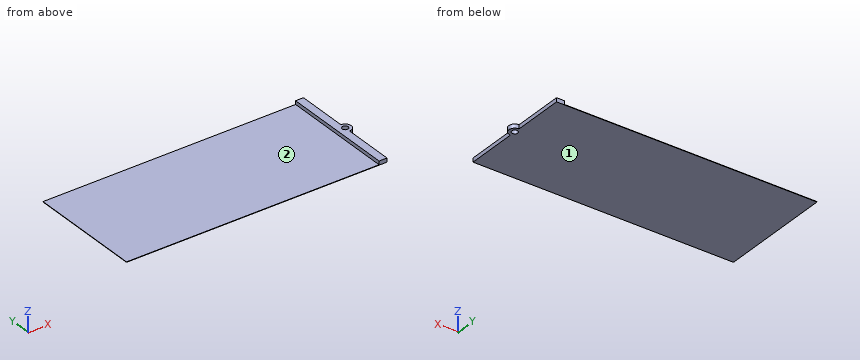
```python
from build123d import *

# Parameters (mm, degrees)
F0_R     = 9.525
F1_DEPTH = 12.7
F2_W     = 812.8
F2_H     = 368.3
F3_DEPTH = 1.27


with BuildPart() as f1:
    # F0 (on Top) → F1 (new body)
    with BuildSketch(Plane.XY):
        with BuildLine():
            Line((-157.734471, -102.348973), (-132.334471, -102.348973))
            Line((-132.334471, -102.348973), (-132.334471, 62.751027))
            ThreePointArc((-132.334471, 62.751027), (-113.284471, 81.801027), (-132.334471, 100.851027))
            Line((-132.334471, 100.851027), (-132.334471, 265.951027))
            Line((-132.334471, 265.951027), (-157.734471, 265.951027))
            Line((-157.734471, 265.951027), (-157.734471, -102.348973))
        make_face()
        with Locations((-132.334471, 81.801027)):
            Circle(F0_R, mode=Mode.SUBTRACT)
    extrude(amount=F1_DEPTH)

    # F2 (on Top) → F3 (join)
    with BuildSketch(Plane.XY):
        with Locations((-564.134471, 81.801027)):
            Rectangle(F2_W, F2_H)
    extrude(amount=F3_DEPTH)


solid = f1.part
```
The listing builds one solid part. Answer for the finished solid, in the listing's coordinates (mm). Face numbers are marked on the shaded views. A direction names the side the tool comes from. Round coordinates to 2 decimals unless told otherwise and drop trailing zeros. Loops run counter-clockwise (first coordinate to the right, second up) from the corner with the lowest first, then second, coordinate; pieces in that order, holes last.
1) A cutting plane is placed at A-A on y = 37.5. Determine the outline of the cut face in (x, z).
Outcome:
outline: (-970.53, 0) - (-132.33, 0) - (-132.33, 12.7) - (-157.73, 12.7) - (-157.73, 1.27) - (-970.53, 1.27) - close
2) A cutting plane is placed at C-C on x = -374. Determine the outline of the cut face in (y, z), plus the area to 3 significant figures.
Outcome:
outline: (-102.35, 0) - (265.95, 0) - (265.95, 1.27) - (-102.35, 1.27) - close
area: 468 mm2
3) Given P1, Ø2, axis at x = -868.5, y = 173, coming from the +Z side; P2, Ø6, axis at x = -595.5, y = -42.5, coming from the -Z side; P3, Ø6, axis at y = 220, z = 4.5, coming from the +X side, each flat-ended and moving along its own axis, determine where each tip first touches the part or whether it passes through.
Outcome:
P1: stops at z = 1.27
P2: stops at z = 0
P3: stops at x = -132.33
4) Consider line 1 (X direction, y = 83, z = 12.25); line 2 (X direction, y = 109.5, z = 12.25); line 3 (Z direction, x = -698, y = 103). Determine where each line is inside the solid, lowest interval first.
Outcome:
line 1: x = -157.73 to -141.78, -122.89 to -113.32
line 2: x = -157.73 to -132.33
line 3: z = 0 to 1.27
5) A cutting plane is placed at B-B on z = 8.5. Determine the outline of the cut face in (x, y) (3 decimals).
Outcome:
outline: (-157.734, -102.349) - (-132.334, -102.349) - (-132.334, 62.751) arc R19.05 ccw to (-132.334, 100.851) - (-132.334, 265.951) - (-157.734, 265.951) - close; hole circle Ø19.05 at (-132.334, 81.801)
6) For the marked faces 1 and 2, determine the directions among +Z, -Z, +X, -X, +Y, -Y from which every point of the face is accessible in a straight line to the end or side of a thin tool.
Outcome:
face 1: -Z, +X, -X, +Y, -Y
face 2: +Z, -X, +Y, -Y
